Geometry check sheet. Reference: drawing and pictorial views, mm from the part's lowest x, y, z. A direction names the side the tool comes from. Give positions to 0.01 mm unless a question says otherwise; leave off trailing zeros. Write each loop counter-clockwise with the first axis right and the second up, starting at its lowest first coordinate (ties: lowest second). Pieces come first, ordered by that corner, then holes. Notation, with made-up numbers: (82, -21) - (111, -21) arc R21 ccw to (111, -15) - close; hole circle Ø11 at (48, 3). An arc over 180 degrees is marked (long way). Write item = value, one per line. Start each with the question number.
(1) Thickness scan on L1, parallel to X at y = 0.1, z = 3; L2, parallel to X at y = 0.7, z = 3; L3, parallel to Z at x = 0.75, y = 0.2. Record the ranges inside material, lowest first.
(2) Draft check along Z on the marked faces 3, 4 and 5. Enter one of: pulls with the +Z half, pulls with the -Z half, needs draft (parallel to the pull), parting line crosses it, or undercut.
(3) Access from +Z, -Z, +X, -X, +Y, -Y to the whole of each face (thin tool, end or side, straight path). Record for the marked faces 1 and 2.
(4) Section check B-B, the plane z = 3. Enter the section's corners in (x, y).
(5) Section check D-D, the plane y = 2.15. Enter the section's corners in (x, z), plus the area to 3 significant figures.
(6) Section check A-A, the plane x = 3. Enter the section's corners in (y, z).
(7) Section check C-C, the plane z = 5.4. Enter the section's corners in (x, y), plus the area to 3 significant figures.
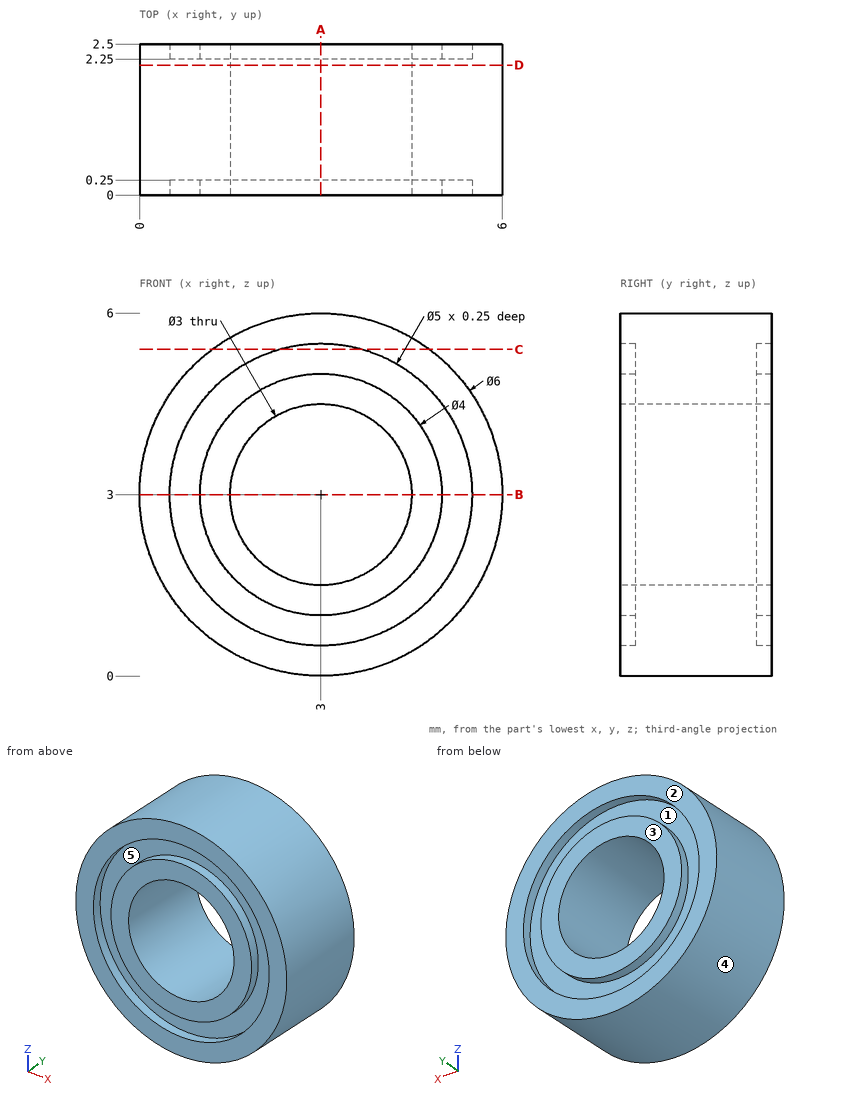
Model answer:
q1.L1 = 0 to 0.5, 1 to 1.5, 4.5 to 5, 5.5 to 6
q1.L2 = 0 to 1.5, 4.5 to 6
q1.L3 = 1.02 to 1.91, 4.09 to 4.98
q2.face_3 = needs draft
q2.face_4 = parting line crosses it
q2.face_5 = undercut
q3.face_1 = +Y
q3.face_2 = +Z, -Z, +X, -X, +Y
q4.outline = (0, 0) - (0.5, 0) - (0.5, 0.25) - (1, 0.25) - (1, 0) - (1.5, 0) - (1.5, 2.5) - (1, 2.5) - (1, 2.25) - (0.5, 2.25) - (0.5, 2.5) - (0, 2.5) - close; (4.5, 0) - (5, 0) - (5, 0.25) - (5.5, 0.25) - (5.5, 0) - (6, 0) - (6, 2.5) - (5.5, 2.5) - (5.5, 2.25) - (5, 2.25) - (5, 2.5) - (4.5, 2.5) - close
q5.outline = circle Ø6 at (3, 3); hole circle Ø3 at (3, 3)
q5.area = 21.2 mm²
q6.outline = (0, 0) - (2.5, 0) - (2.5, 0.5) - (2.25, 0.5) - (2.25, 1) - (2.5, 1) - (2.5, 1.5) - (0, 1.5) - (0, 1) - (0.25, 1) - (0.25, 0.5) - (0, 0.5) - close; (0, 4.5) - (2.5, 4.5) - (2.5, 5) - (2.25, 5) - (2.25, 5.5) - (2.5, 5.5) - (2.5, 6) - (0, 6) - (0, 5.5) - (0.25, 5.5) - (0.25, 5) - (0, 5) - close
q7.outline = (1.2, 0) - (2.3, 0) - (2.3, 0.25) - (3.7, 0.25) - (3.7, 0) - (4.8, 0) - (4.8, 2.5) - (3.7, 2.5) - (3.7, 2.25) - (2.3, 2.25) - (2.3, 2.5) - (1.2, 2.5) - close
q7.area = 8.30 mm²
